Can you work these out from the model? Positions are in its coordinate system, mm. Face numbers are marked on the shaded views. A direction names the side the tool comes from. Round coordinates to 2 decimals unless told otherwise and drop trailing zeros. Write each loop counter-clockwise with the first axis right and the second up, starting at its lowest first coordinate (ties: lowest second). Pieces come first, ordered by that corner, then holes.
Q1. We'd pull the mould along X, two halves only. Please class the marked faces 4, 5 and 6: +X half, -X half, draft (parallel to the pull), parting line (faces both ways), or undercut.
Q2. For the marked faces 1, 2 and 3, which set-ups out of +Z, -Z, +X, -X, +Y, -Y let a thin tool reach every point of the face, with its end or its side?
Q3. If we section it at B-B (x = -8): Please give me the cut outline in (y, z).
Q4. If we section it at D-D (x = 1.75): Please give me the cut outline in (y, z), plus the area to 3 significant figures.
Q5. If we section it at C-C (y = -0.35): Please give me the cut outline in (x, z).
Q6. Please list where these lines run through material, in increasing order: line 1 along Z through (x, y) = (6, -1.05); line 2 along Z through (x, y) = (-6, -1.9); line 3 along X through (y, z) = (-1, -8.75).
Q7. I'm going to push a flat-ended pin straight in: pin 1 Ø0.9 at (x, y) = (-6, -1.5) entering from +Z. Where does the tip first touch, or does it pass through?
from build123d import *

# Parameters (mm, degrees)
F2_DEPTH = 2.9
F3_R     = 1.44999
F4_D     = 0.3


# Not quite as in the source:
# - a fillet or chamfer is up to 0.001 mm smaller than in the source, because OpenCascade refuses the exact size


with BuildPart() as f2:
    # F0 (on Front) → F2 (new body)
    with BuildSketch(Plane.XZ):
        Polygon((9.0052141035, -8.636), (0, -8.636), (0, -9.936), (-3.7947858965, -9.936), (-10.4947858965, -9.936), (-10.4947858965, -8.636), (-17.9947858965, -8.636), (-17.9947858965, -11.236), (9.0052141035, -11.236), align=None)
        with BuildLine():
            Line((0, -9.936), (0, -8.636))
            ThreePointArc((0, -8.636), (-3.9876610239, -7.6602255553), (-7.0741970545, -4.9534061043))
            Line((-7.0741970545, -4.9534061043), (-8.7125011431, -6.100558977))
            ThreePointArc((-8.7125011431, -6.100558977), (-6.5410785986, -8.3868222091), (-3.7947858965, -9.936))
            Line((-3.7947858965, -9.936), (0, -9.936))
        make_face()
    extrude(amount=F2_DEPTH)

    # F3 (radius 1.45 in the source; OpenCascade refuses exactly that, so slightly less here)
    f3_edges = [f2.edges().sort_by_distance(p)[0] for p in [
        (9.005214, -2.9, -9.936),
        (9.005214, 0, -9.936),
        (-17.994786, -2.9, -9.936),
        (-17.994786, 0, -9.936),
    ]]
    fillet(f3_edges, radius=F3_R)

    # F4 (through all)
    with Locations(Plane(origin=(0, 0, 0), x_dir=(1, 0, 0), z_dir=(0, 1, 0))):
        with Locations((-3.7947858965, 9.936)):
            Hole(F4_D / 2)


solid = f2.part
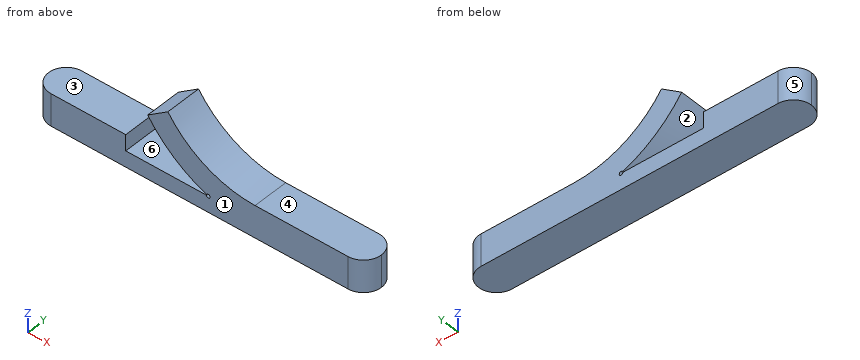
A:
1. face 4: draft
1. face 5: -X half
1. face 6: undercut
2. face 1: +Z, -Z, +X, -X, -Y
2. face 2: +Y, -Y
2. face 3: +Z, -X, +Y, -Y
3. outline: (-2.9, -11.24) - (0, -11.24) - (0, -9.94) - (-2.9, -9.94) - close; (-2.9, -7.01) - (0, -7.01) - (0, -5.6) - (-2.9, -5.6) - close
4. outline: (-2.9, -11.24) - (0, -11.24) - (0, -8.64) - (-2.9, -8.64) - close
4. area: 7.54 mm2
5. outline: (-17.49, -11.24) - (8.5, -11.24) - (8.5, -8.64) - (0, -8.64) arc R8.64 cw to (-7.07, -4.95) - (-8.71, -6.1) arc R10.64 ccw to (-3.93, -9.88) arc R0.15 cw (long way) to (-3.94, -9.94) - (-10.49, -9.94) - (-10.49, -8.64) - (-17.49, -8.64) - close
6. line 1: z = -11.24 to -8.64
6. line 2: z = -11.24 to -9.94, -8.78 to -6.21
6. line 3: x = -17.92 to -10.49, -6.05 to 8.93
7. pin 1: stops at z = -5.74
